Input: dimensioned drawing with shaded views. Units: mm. Origin: part minimum x, y, z. Round coordinates to 2 decimals unless told otherwise and drop trailing zeros. Write each loop counter-clockwise with the first axis right and the second up, starting at its lowest first coordinate (ties: lowest second). Pieces come first, ordered by that corner, then holes. Notation, with made-up numbers: (62.5, -30) -> (112.5, -30) arc R30 cw to (112.5, 4) -> close; hole circle Ø7 at (52, 58). An arc over 180 degrees is marked (long way). One line per item, written item: value. Start each with the question number.
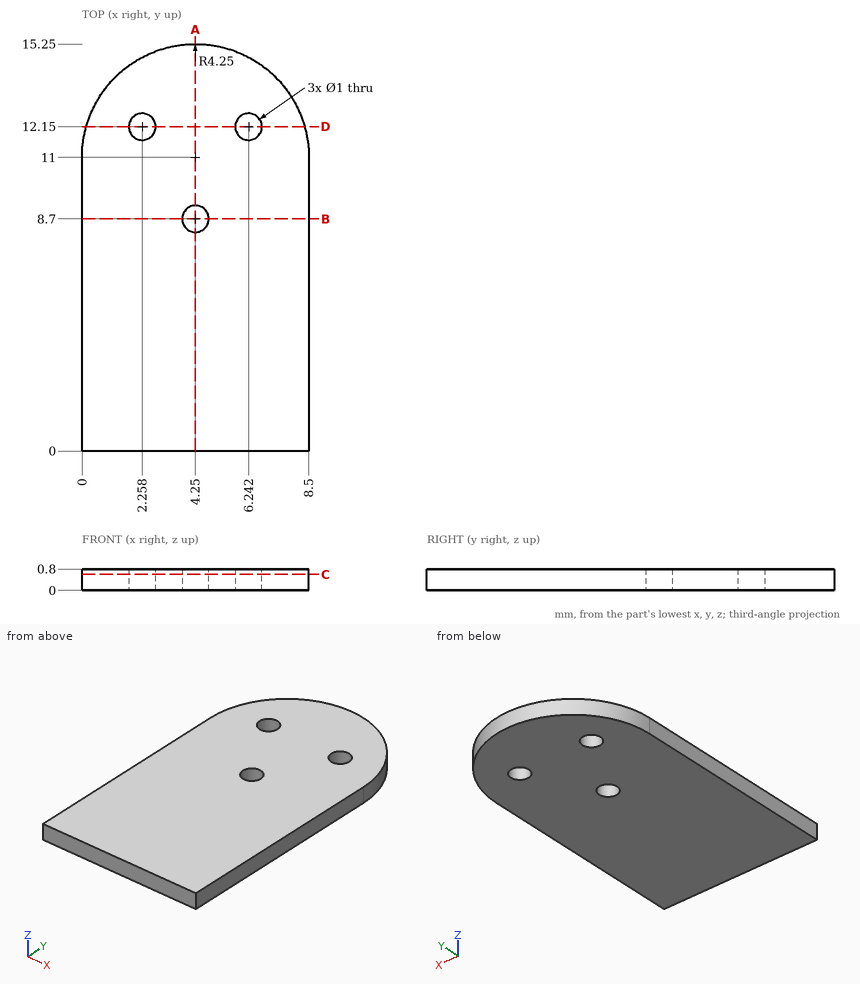
(1) Section query D-D (y = 12.15). Output: boundary loops of the cut face in (x, z).
(2) Section query C-C (z = 0.6). Output: boundary loops of the cut face in (x, y), and give its area (3 significant figures).
(3) Section query A-A (x = 4.25). Output: boundary loops of the cut face in (y, z).
(4) Section query B-B (y = 8.7). Output: boundary loops of the cut face in (x, z).
(5) Pin query (flat end, axial travel): pin 1 (3 mm diameter, centred on x = 6.5, y = 2, fed in from -Z). Return the tip coordinate at first contact, or that it passes through.
(6) Line query: probe 1 along Y at (x, z) = (4.25, 0.6); probe 2 along Y at (x, z) = (4, 0.2); probe 3 along Y at (x, z) = (7, 0.6). Output: solid intervals per line, ascending.
Results list:
1. outline: (0.16, 0) -> (1.76, 0) -> (1.76, 0.8) -> (0.16, 0.8) -> close; (2.76, 0) -> (5.74, 0) -> (5.74, 0.8) -> (2.76, 0.8) -> close; (6.74, 0) -> (8.34, 0) -> (8.34, 0.8) -> (6.74, 0.8) -> close
2. outline: (0, 0) -> (8.5, 0) -> (8.5, 11) arc R4.25 ccw to (0, 11) -> close; hole circle Ø1 at (2.26, 12.15); hole circle Ø1 at (4.25, 8.7); hole circle Ø1 at (6.24, 12.15)
2. area: 120 mm^2
3. outline: (0, 0) -> (8.2, 0) -> (8.2, 0.8) -> (0, 0.8) -> close; (9.2, 0) -> (15.25, 0) -> (15.25, 0.8) -> (9.2, 0.8) -> close
4. outline: (0, 0) -> (3.75, 0) -> (3.75, 0.8) -> (0, 0.8) -> close; (4.75, 0) -> (8.5, 0) -> (8.5, 0.8) -> (4.75, 0.8) -> close
5. pin 1: stops at z = 0
6. probe 1: y = 0 to 8.2, 9.2 to 15.25
6. probe 2: y = 0 to 8.27, 9.13 to 15.24
6. probe 3: y = 0 to 14.24
